Part model, mm, in its own coordinate system. A direction names the side the tool comes from. Round coordinates to 2 decimals unless told otherwise and drop trailing zeros. Write each loop counter-clockwise with the first axis right and the second up, starting at its lowest first coordinate (ties: lowest second). Pieces come first, ordered by that corner, then holes. Notation, with made-up numbers: M 87.25,-37 L 106.25,-37 A23 cw 106.25,-2 Z; hole C 75,21 d11. An arc over 180 degrees is marked long. One line per question, with ' | ' between items. Start each with the question number.
1) Saw through at A-A (x = 36.65). List the corners of the cut face in (y, z), plus the area to 3 significant figures.
2) Saw through at B-B (z = 1). List the corners of the cut face in (x, y), plus the area to 3 significant figures.
3) Wall check: probe 1 along X at (y, z) = (-26, 5.15); probe 2 along Z at (x, y) = (5.65, -23.5); probe 3 along Z at (x, y) = (21.15, -24.5). Give the ranges that are in metal, low to high. Write a range as [from, to].
4) Saw through at C-C (x = 19). List the corners of the cut face in (y, z).
5) Drop flat-ended pins along their axis: pin 1 Ø20.5 at (y, z) = (-13.5, -4.5) entering from -X; pin 2 Ø2 at (x, z) = (33.5, -24) entering from +Y; pin 3 Ø2.5 at (x, z) = (36.65, -25.85) entering from +Y; pin 4 Ø16 at (x, y) = (10.5, -13) entering from -Z. Give the stop position or say it passes through.
6) Tool access for faces 1 (the face through (0.986, -12.354, -8.292)), 2 (the face through (21, -6, 8)): list every direction of +Z, -Z, +X, -X, +Y, -Y with a clear straight run to the whole face (end or side of a thin tool).
7) Mould opens along Z. For faces 3 (the face through (38.036, -24.704, 4.575)), 4 (the face through (33.16, -24.7, -15.33)), 5 (the face through (21, -9, 11)), 6 (the face through (30, -21.5, -21)) say: pulls with the +Z half, pulls with the -Z half, needs draft (parallel to the pull), parting line crosses it, or undercut.
8) Saw through at D-D (y = -4). List the corners of the cut face in (x, z), plus the area to 3 significant figures.
```python
from build123d import *

# Parameters (mm, degrees)
BOX009_W          = 44
BOX009_H          = 24
BOX009_DEPTH      = 70
PRISM001_DEPTH    = 2
BOX008_W          = 42.3
BOX008_H          = 38
BOX008_DEPTH      = 3
CYLINDER005_R     = 13
CYLINDER005_DEPTH = 10
CYLINDER002_R     = 1.5
CYLINDER002_DEPTH = 10
CYLINDER003_R     = 1.5
CYLINDER003_DEPTH = 10
CYLINDER004_R     = 1.5
CYLINDER004_DEPTH = 10
CYLINDER001_R     = 1.5
CYLINDER001_DEPTH = 10
BOX007_W          = 42.3
BOX007_H          = 6.5
BOX007_DEPTH      = 42.3
BOX010_W          = 44
BOX010_H          = 24
BOX010_DEPTH      = 70
PRISM002_DEPTH    = 2


with BuildPart() as cube009:
    # Box009 → Box009 (new body)
    with BuildSketch(Plane(origin=(0, -43, -25.5), x_dir=(1, 0, 0), z_dir=(0, 0, 1))):
        with Locations((22, 12)):
            Rectangle(BOX009_W, BOX009_H)
    extrude(amount=BOX009_DEPTH)


with BuildPart() as cut012:
    # Prism001 → Prism001 (new body)
    with BuildSketch(Plane(origin=(0, -19, 2), x_dir=(0, 0, -1), z_dir=(1, 0, 0))):
        Polygon((23, 0), (-11.5, 19.918584), (-11.5, -19.918584), align=None)
    extrude(amount=PRISM001_DEPTH)

    # Cut012: cut Cube009
    add(cube009.part, mode=Mode.SUBTRACT)


with BuildPart() as cut012_1:
    # Cut012 placement: moved
    add(cut012.part.moved(Location((0, -3, -4))))


with BuildPart() as cube008:
    # Box008 → Box008 (new body)
    with BuildSketch(Plane(origin=(0, -28, 8), x_dir=(1, 0, 0), z_dir=(0, 0, 1))):
        with Locations((21.15, 19)):
            Rectangle(BOX008_W, BOX008_H)
    extrude(amount=BOX008_DEPTH)


with BuildPart() as cylinder005:
    # Cylinder005 → Cylinder005 (new body)
    with BuildSketch(Plane(origin=(21.15, -14, 21.15), x_dir=(1, 0, 0), z_dir=(0, -1, 0))):
        Circle(CYLINDER005_R)
    extrude(amount=CYLINDER005_DEPTH)


with BuildPart() as cylinder002:
    # Cylinder002 → Cylinder002 (new body)
    with BuildSketch(Plane(origin=(5.65, -14, 36.65), x_dir=(1, 0, 0), z_dir=(0, -1, 0))):
        Circle(CYLINDER002_R)
    extrude(amount=CYLINDER002_DEPTH)


with BuildPart() as cylinder003:
    # Cylinder003 → Cylinder003 (new body)
    with BuildSketch(Plane(origin=(36.65, -14, 5.65), x_dir=(1, 0, 0), z_dir=(0, -1, 0))):
        Circle(CYLINDER003_R)
    extrude(amount=CYLINDER003_DEPTH)


with BuildPart() as cylinder004:
    # Cylinder004 → Cylinder004 (new body)
    with BuildSketch(Plane(origin=(36.65, -14, 36.65), x_dir=(1, 0, 0), z_dir=(0, -1, 0))):
        Circle(CYLINDER004_R)
    extrude(amount=CYLINDER004_DEPTH)


with BuildPart() as cylinder001:
    # Cylinder001 → Cylinder001 (new body)
    with BuildSketch(Plane(origin=(5.65, -14, 5.65), x_dir=(1, 0, 0), z_dir=(0, -1, 0))):
        Circle(CYLINDER001_R)
    extrude(amount=CYLINDER001_DEPTH)


with BuildPart() as fusion002:
    # Box007 → Box007 (new body)
    with BuildSketch(Plane(origin=(0, -21, 0), x_dir=(1, 0, 0), z_dir=(0, 0, 1))):
        with Locations((21.15, 3.25)):
            Rectangle(BOX007_W, BOX007_H)
    extrude(amount=BOX007_DEPTH)

    # Cut007: cut Cylinder001
    add(cylinder001.part, mode=Mode.SUBTRACT)

    # Cut008: cut Cylinder004
    add(cylinder004.part, mode=Mode.SUBTRACT)

    # Cut009: cut Cylinder003
    add(cylinder003.part, mode=Mode.SUBTRACT)

    # Cut010: cut Cylinder002
    add(cylinder002.part, mode=Mode.SUBTRACT)

    # Cut011: cut Cylinder005
    add(cylinder005.part, mode=Mode.SUBTRACT)


with BuildPart() as fusion002_1:
    # Cut011 placement: moved
    add(fusion002.part.moved(Location((0, -7, -31.5))))

    # Fusion001: union Cube008
    add(cube008.part)

    # Fusion002: union Cut012
    add(cut012_1.part)


with BuildPart() as cube010:
    # Box010 → Box010 (new body)
    with BuildSketch(Plane(origin=(0, -43, -25.5), x_dir=(1, 0, 0), z_dir=(0, 0, 1))):
        with Locations((22, 12)):
            Rectangle(BOX010_W, BOX010_H)
    extrude(amount=BOX010_DEPTH)


with BuildPart() as obj1:
    # Prism002 → Prism002 (new body)
    with BuildSketch(Plane(origin=(0, -19, 2), x_dir=(0, 0, -1), z_dir=(1, 0, 0))):
        Polygon((23, 0), (-11.5, 19.918584), (-11.5, -19.918584), align=None)
    extrude(amount=PRISM002_DEPTH)

    # Cut013: cut Cube010
    add(cube010.part, mode=Mode.SUBTRACT)


with BuildPart() as obj1_1:
    # Cut013 placement: moved
    add(obj1.part.moved(Location((40.3, -3, -4))))

    # Fusion003: union Fusion002
    add(fusion002_1.part)


solid = obj1_1.part
```
Answer key:
1) outline: M -28,-31.5 L -21.5,-31.5 L -21.5,-27.35 L -28,-27.35 Z; M -28,-24.35 L -21.5,-24.35 L -21.5,3.65 L -28,3.65 Z; M -28,6.65 L -21.5,6.65 L -21.5,8 L 10,8 L 10,11 L -28,11 Z | area: 332 mm2
2) outline: M 0,-28 L 14.81,-28 L 14.81,-21.5 L 2,-21.5 L 2,-6.99 L 0,-6.99 Z; M 27.49,-28 L 42.3,-28 L 42.3,-6.99 L 40.3,-6.99 L 40.3,-21.5 L 27.49,-21.5 Z | area: 251 mm2
3) probe 1: x = [0, 4.15], [7.15, 35.15], [38.15, 42.3] | probe 2: z = [-31.5, -27.35], [-24.35, 3.65], [6.65, 11] | probe 3: z = [-31.5, -23.35], [2.65, 11]
4) outline: M -28,-31.5 L -21.5,-31.5 L -21.5,-23.17 L -28,-23.17 Z; M -28,2.47 L -21.5,2.47 L -21.5,8 L 10,8 L 10,11 L -28,11 Z
5) pin 1: stops at x = 0 | pin 2: stops at y = -21.5 | pin 3: passes through | pin 4: stops at z = 8
6) face 1: -Z, +X, -X, +Y | face 2: -Z, +Y
7) face 3: undercut | face 4: undercut | face 5: pulls with the +Z half | face 6: needs draft
8) outline: M 0,6.18 L 2,6.18 L 2,8 L 40.3,8 L 40.3,6.18 L 42.3,6.18 L 42.3,11 L 0,11 Z | area: 134 mm2
